Job drawing, mm, ordinate dimensions from the low corner. One solid piece. A direction names the side the tool comes from. Give positions to 0.01 mm unless a question says otherwise; leave off trailing zeros. Order: outer loops, then holes, each group sorted by start corner. A loop starts at its lowest first (then second) coordinate and runs counter-clockwise, first axis right, second up. Notation, with made-up numbers: (-20.75, 0) - (6.25, 0) arc R34 ccw to (6.25, 30) - close; hole circle Ø5 at (-34.5, 11). An arc over 180 degrees is marked (long way). Write each question's results on one line, items separated by ' | '. Start each with the question number.
1) Drop flat-ended pins along their axis: pin 1 Ø1.5 at (y, z) = (8, 16.5) entering from +X; pin 2 Ø1.5 at (y, z) = (2.5, 12.5) entering from +X; pin 3 Ø5 at (x, y) = (7.5, 10) entering from +Z. Give the stop position or say it passes through.
2) Drill centre lines: line 1 along Y through (x, z) = (17, 12.5); line 2 along Z through (x, y) = (10, 8). Where is each one in solid material? Low to high. Write a range as from..to.
3) Cut at C-C on y = 10. List the corners of the cut face in (x, z).
4) Cut at B-B on x = 10. List the corners of the cut face in (y, z), plus the area to 3 significant figures.
5) Two-plate mould, pull along X, no slides. Class the marked faces 3 and 4: +X half, -X half, draft (parallel to the pull), parting line (faces both ways), or undercut.
6) Cut at D-D on y = 2.5. List the corners of the cut face in (x, z).
7) Cut at A-A on z = 10. List the corners of the cut face in (x, y).
8) Tool access for the marked faces 1 and 2: list every direction of +Z, -Z, +X, -X, +Y, -Y with a clear straight run to the whole face (end or side of a thin tool).
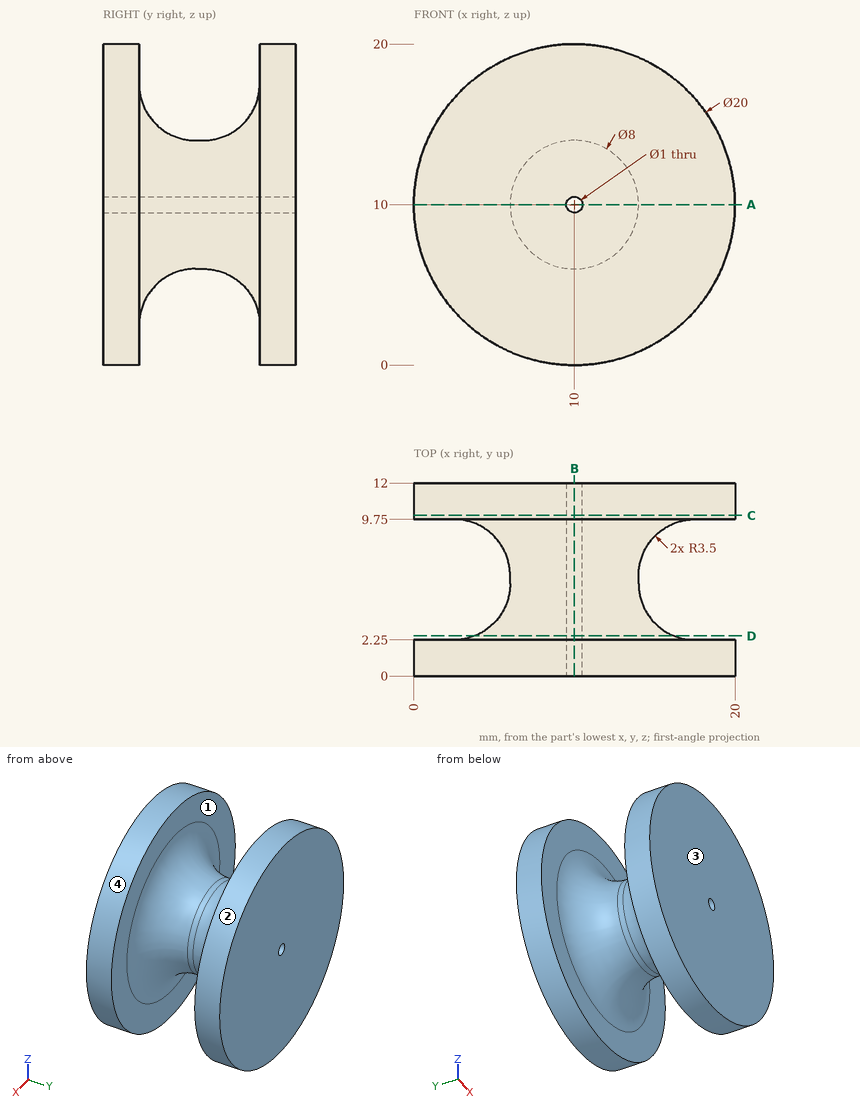
Results:
1) pin 1: through | pin 2: x = 19.84 | pin 3: z = 20
2) line 1: 0..2.25, 9.75..12 | line 2: 5.53..9.5, 10.5..14.47
3) outline: circle Ø20 at (10, 10); hole circle Ø1 at (10, 10)
4) outline: (0, 0) - (2.25, 0) - (2.25, 2.5) arc R3.5 cw to (5.75, 6) - (6.25, 6) arc R3.5 cw to (9.75, 2.5) - (9.75, 0) - (12, 0) - (12, 9.5) - (0, 9.5) - close; (0, 10.5) - (12, 10.5) - (12, 20) - (9.75, 20) - (9.75, 17.5) arc R3.5 cw to (6.25, 14) - (5.75, 14) arc R3.5 cw to (2.25, 17.5) - (2.25, 20) - (0, 20) - close | area: 149 mm^2
5) face 3: draft | face 4: parting line
6) outline: circle Ø12.4 at (10, 10); hole circle Ø1 at (10, 10)
7) outline: (0, 0) - (9.5, 0) - (9.5, 12) - (0, 12) - (0, 9.75) - (2.5, 9.75) arc R3.5 cw to (6, 6.25) - (6, 5.75) arc R3.5 cw to (2.5, 2.25) - (0, 2.25) - close; (10.5, 0) - (20, 0) - (20, 2.25) - (17.5, 2.25) arc R3.5 cw to (14, 5.75) - (14, 6.25) arc R3.5 cw to (17.5, 9.75) - (20, 9.75) - (20, 12) - (10.5, 12) - close
8) face 1: none | face 2: +Y, -Y
